The drawing under review shows one solid part. Ordinate dimensions are in mm from its lowest x, y, z. A direction names the side the tool comes from. Coordinates: 2 decimals unless noted, no trailing zeros. Order: outer loops, then holes, each group sorted by start corner. A loop starts at its lowest first (then second) coordinate and runs counter-clockwise, first axis right, second up. Notation, with made-up numbers: (76.5, 19.5) -> (105.5, 19.5) arc R11 cw to (105.5, 23.5) -> close; hole circle Ø6 at (23.25, 16). An arc over 180 degrees is marked (long way). Write item = value, one per line.
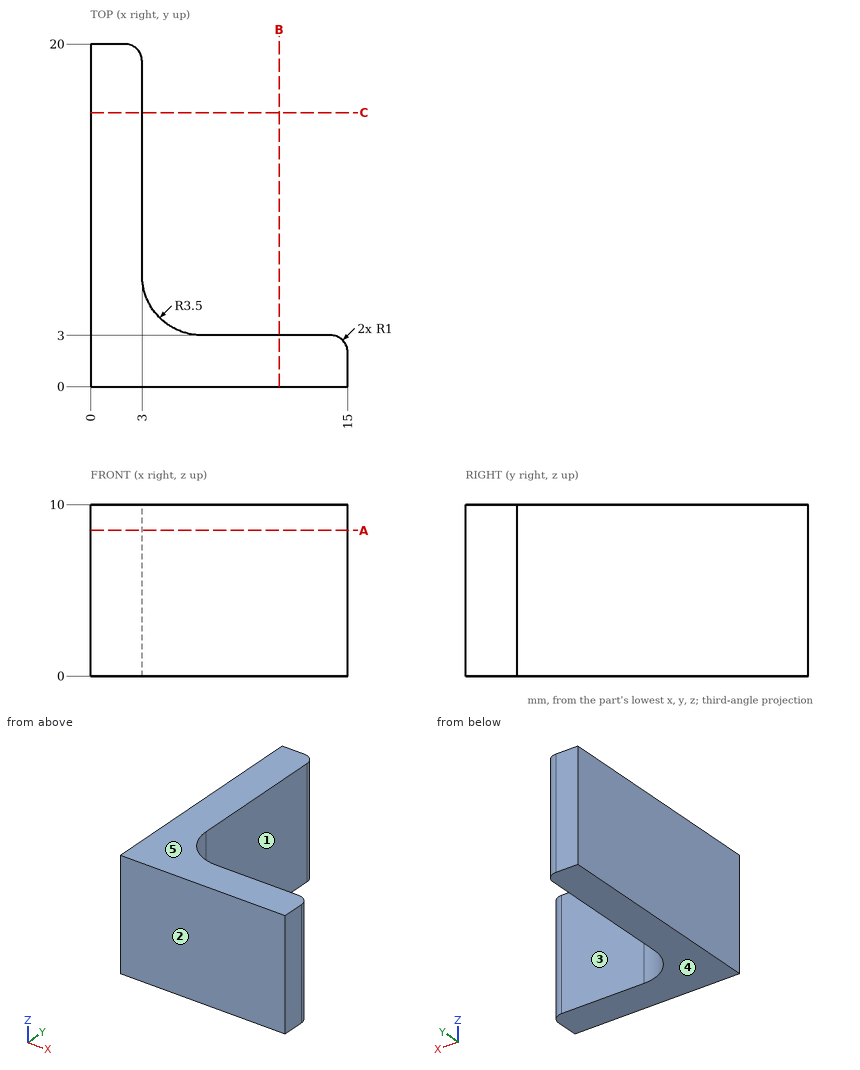
(1) Insertion check: pin 1 (5 mm diameter, centred on y = 13, z = 7.5, fed in from +X); pin 2 (2 mm diameter, centred on x = 12, z = 6, fed in from +Y). Each pin has a flat end and moves straight along its axis. Give the tip position at first contact, or say it passes through.
Report:
pin_1 = 3
pin_2 = 3
(2) For the marked faces 1 and 2, list the 3-axis set-ups (+Z, -Z, +X, -X, +Y, -Y) from which the entire face can be reached by the end or side of a thin tool; tool diameter is ignored.
Report:
face_1 = +Z, -Z, +X, +Y
face_2 = +Z, -Z, +X, -X, -Y
(3) We need section A-A (z = 8.5). Write out the cut boundary in (x, y), and give its area (3 significant figures).
Report:
outline = (0, 0) -> (15, 0) -> (15, 2) arc R1 ccw to (14, 3) -> (6.5, 3) arc R3.5 cw to (3, 6.5) -> (3, 19) arc R1 ccw to (2, 20) -> (0, 20) -> close
area = 98.2 mm²
(4) The part is to be moulded in two halves that separate along Z. For the marked faces 3, 4 and 5, say which applies: released by +Z, released by -Z, zero draft, split by the parting line, or undercut.
Report:
face_3 = zero draft
face_4 = released by -Z
face_5 = released by +Z
(5) For L1, parallel to Y at x = 7, z = 8.75; L2, parallel to X at y = 5.25, z = 1.5, list the stretches that pass through material, from the lowest coordinate up.
Report:
L1 = 0 to 3
L2 = 0 to 3.23
(6) We need section B-B (x = 11). Write out the cut boundary in (y, z), and give its area (3 significant figures).
Report:
outline = (0, 0) -> (3, 0) -> (3, 10) -> (0, 10) -> close
area = 30.0 mm²
